from build123d import *

# Parameters (mm, degrees)
EXTRUDE_1_DEPTH     = 11
CUT_EXTRUDE_1_DEPTH = 15
SKETCH_3_R          = 9
EXTRUDE_2_DEPTH     = 20
SKETCH_4_W          = 40
SKETCH_4_H          = 27
CUT_EXTRUDE_2_DEPTH = 1
SKETCH_6_R          = 5.5
CUT_EXTRUDE_3_DEPTH = 76.048317769
EXTRUDE_3_DEPTH     = 26
FILLET_1_R          = 13
FILLET_2_R          = 5
CUT_EXTRUDE_4_DEPTH = 10


with BuildPart() as part:
    # 스케치1 → 보스-돌출1 (new body)
    with BuildSketch(Plane.XY):
        with BuildLine():
            Line((-67, 13.5), (0, 13.5))
            ThreePointArc((0, 13.5), (13.5, 0), (0, -13.5))
            Line((0, -13.5), (-67, -13.5))
            Line((-67, -13.5), (-67, 13.5))
        make_face()
    extrude(amount=EXTRUDE_1_DEPTH)

    # 스케치2 → 컷-돌출1 (cut)
    with BuildSketch(Plane.XY.offset(11)):
        with BuildLine():
            Line((-54, 4), (-41, 4))
            ThreePointArc((-41, 4), (-37, 0), (-41, -4))
            Line((-41, -4), (-54, -4))
            ThreePointArc((-54, -4), (-58, 0), (-54, 4))
        make_face()
    extrude(amount=-CUT_EXTRUDE_1_DEPTH, mode=Mode.SUBTRACT)

    # 스케치3 → 보스-돌출2 (add)
    with BuildSketch(Plane.XY.offset(11)):
        Circle(SKETCH_3_R)
    extrude(amount=EXTRUDE_2_DEPTH)

    # 스케치4 → 컷-돌출2 (cut)
    with BuildSketch(Plane.XY.offset(11)):
        with Locations((-47, 0)):
            Rectangle(SKETCH_4_W, SKETCH_4_H)
    cut_extrude_2 = extrude(amount=-CUT_EXTRUDE_2_DEPTH, mode=Mode.SUBTRACT)

    # 대칭 복사1: 컷-돌출2 across plane
    add(cut_extrude_2.mirror(Plane.XY.offset(5.5)), mode=Mode.SUBTRACT)

    # 스케치6 → 컷-돌출3 (cut, through all)
    with BuildSketch(Plane.XY.offset(31)):
        Circle(SKETCH_6_R)
    extrude(amount=-CUT_EXTRUDE_3_DEPTH, mode=Mode.SUBTRACT)

    # 스케치8 → 보스-돌출3 (add)
    with BuildSketch(Plane.XY.offset(31)):
        Polygon((48.267141866, 52.030952398), (3.01230787, 6.776118402), (7.254948557, 2.533477715), (52.509782553, 47.788311711), align=None)
    extrude(amount=-EXTRUDE_3_DEPTH)

    # 필렛1
    fillet_1_edges = [part.edges().sort_by_distance(p)[0] for p in [
        (50.38846221, 49.909632055, 31),
        (50.38846221, 49.909632055, 5),
    ]]
    fillet(fillet_1_edges, radius=FILLET_1_R - 0.0001)  # a hair under: the kernel refuses the full size

    # 필렛2
    fillet_2_edges = [part.edges().sort_by_distance(p)[0] for p in [
        (-67, -13.5, 5.5),
        (-67, 13.5, 5.5),
    ]]
    fillet(fillet_2_edges, radius=FILLET_2_R)

    # 스케치11 → 컷-돌출4 (cut)
    with BuildSketch(Plane(origin=(2.360735421, -2.360735421, 0), x_dir=(0, 0, -1), z_dir=(0.7071067811865477, -0.7071067811865475, 0))):
        with BuildLine():
            Line((-14, 58), (-14, 30))
            ThreePointArc((-14, 30), (-18, 26), (-22, 30))
            Line((-22, 30), (-22, 58))
            ThreePointArc((-22, 58), (-18, 62), (-14, 58))
        make_face()
    extrude(amount=-CUT_EXTRUDE_4_DEPTH, mode=Mode.SUBTRACT)


solid = part.part
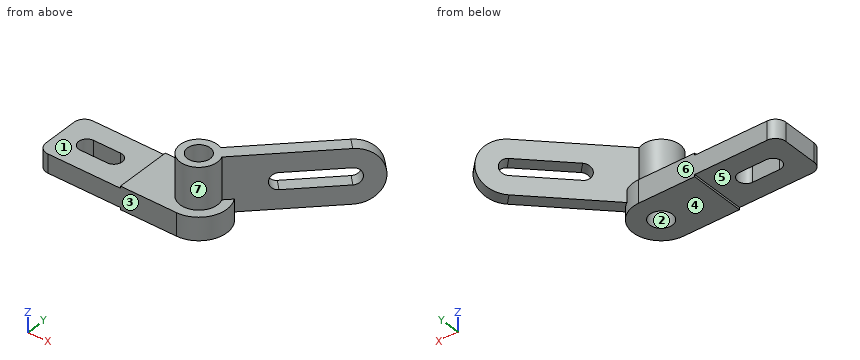
Input: part model. Units: mm. Frame: model coordinates. Face numbers are marked on the shaded views. A direction names the side the tool comes from. Round coordinates to 2 decimals unless told otherwise and drop trailing zeros. Order: outer loops, then holes, each group sorted by start corner. A loop starts at its lowest first (then second) coordinate and runs counter-clockwise, first axis right, second up.
1. Set-up query: the marked faces 4, 5, 6 and 7. Return all of +Z, -Z, +X, -X, +Y, -Y with unobstructed straight access to the full face (end or side cutting, diameter ignored); none if empty.
The answers:
face 4: -Z, +X, -X, +Y, -Y
face 5: -Z, -X, +Y, -Y
face 6: +Z, -Z, -X, +Y
face 7: +Z
2. Cut plane B-B, the plane x = -42.5. Output: boundary loops of the cut face in (y, z).
The answers:
outline: (-13.5, 1) - (-4, 1) - (-4, 10) - (-13.5, 10) - close; (4, 1) - (13.5, 1) - (13.5, 10) - (4, 10) - close
3. Material intervals for line 1 (Y direction, x = 0, z = 18); line 2 (X direction, y = 1, z = 23); line 3 (Y direction, x = 1.5, z = 10), sorted ascending.
The answers:
line 1: y = -9 to -5.5, 5.5 to 9
line 2: x = -8.94 to -5.41, 5.41 to 8.94
line 3: y = -13.42 to -5.29, 5.29 to 13.42
4. Cut plane C-C, the plane y = 29. Output: boundary loops of the cut face in (x, z), then the cut area to 3 significant figures.
The answers:
outline: (25.24, 5) - (33.72, 5) - (33.72, 14) - (25.24, 14) - close; (25.24, 22) - (33.72, 22) - (33.72, 31) - (25.24, 31) - close
area: 153 mm2
5. Cut plane A-A, the plane y = 0. Output: boundary loops of the cut face in (x, z).
The answers:
outline: (-67, 1) - (-58, 1) - (-58, 10) - (-67, 10) - close; (-37, 1) - (-27, 1) - (-27, 0) - (-5.5, 0) - (-5.5, 31) - (-9, 31) - (-9, 11) - (-27, 11) - (-27, 10) - (-37, 10) - close; (5.5, 0) - (13.5, 0) - (13.5, 11) - (9, 11) - (9, 31) - (5.5, 31) - close
6. Pin query (flat end, axial travel): P1, Ø8, axis at x = 11.5, z = 22.5, coming from the +Y side; P2, Ø8, axis at x = -49, y = -5, coming from the +Z side; P3, Ø8, axis at x = -42.5, y = -6, coming from the -Z side. Return the tip coordinate at first contact, or that it passes through.
The answers:
P1: stops at y = 19.26
P2: stops at z = 10
P3: stops at z = 1
7. Mould query, pull axis Y, two halves, no side actions, for the marked faces 1, 2 and 3. Classes: released by +Y, released by -Y, zero draft, split by the parting line, or undercut.
The answers:
face 1: zero draft
face 2: undercut
face 3: released by -Y
8. Cut plane D-D, the plane z = 23.5. Output: boundary loops of the cut face in (x, y).
The answers:
outline: (4.2, 7.96) arc R9 ccw (long way) to (8.27, 3.55) - (51.65, 46.93) - (47.4, 51.17) - close; hole circle Ø11 at (0, 0)
